Autodesk Inventor part; units mm, degrees
ref_plane "YZ Plane" through (0, 0, 0) normal (1, 0, 0) x (0, 1, 0)
ref_plane "XZ Plane" through (0, 0, 0) normal (0, 1, 0) x (-1, 0, 0)
ref_plane "XY Plane" through (0, 0, 0) normal (0, 0, 1) x (1, 0, 0)
sketch "Sketch1" plane through (0, 0, 0) normal (0, 1, 0) x (-1, 0, 0)
  line L0 (0, 0) -> (0, -11.938)
  line L1 (-15.24, 3.3655) -> (-15.24, -15.3035)
  line L2 (0, 0) -> (-15.24, 3.3655)
  line L3 (0, -11.938) -> (-15.24, -15.3035)
  line L4 (-15.24, 3.3655) -> (-19.05, 3.3655)
  line L5 (-19.05, 3.3655) -> (-19.05, 2.0955)
  line L6 (-19.05, 2.0955) -> (-15.24, 2.0955)
  line L7 (-15.24, 2.0955) -> (-15.24, 3.3655)
  line L8 (-15.24, -15.3035) -> (-19.05, -15.3035)
  line L9 (-19.05, -15.3035) -> (-19.05, -14.0335)
  line L10 (-19.05, -14.0335) -> (-15.24, -14.0335)
  line L11 (-15.24, -14.0335) -> (-15.24, -15.3035)
  line L12 (0, 0) -> (0, 3.175)
  line L13 (-15.24, 3.3655) -> (-15.24, 6.5405)
  line L14 (0, -11.938) -> (0, -15.113)
  line L15 (-15.24, -15.3035) -> (-15.24, -18.4785)
  line L16 (-15.24, -18.4785) -> (0, -15.113)
  line L17 (0, 3.175) -> (-15.24, 6.5405)
  line L18 (-15.24, 6.5405) -> (-34.29, 6.5405)
  line L19 (-19.05, 3.3655) -> (-34.29, 3.3655)
  line L20 (-34.29, 3.3655) -> (-34.29, 6.5405)
  line L21 (-15.24, -18.4785) -> (-34.29, -18.4785)
  line L22 (-34.29, -18.4785) -> (-34.29, -15.3035)
  line L23 (-34.29, -15.3035) -> (-19.05, -15.3035)
  line L24 (-34.29, 6.5405) -> (-37.465, 6.5405)
  line L25 (-37.465, 6.5405) -> (-37.465, -18.4785)
  line L26 (-37.465, -18.4785) -> (-34.29, -18.4785)
  line L27 (-34.29, -18.4785) -> (-34.29, 6.5405)
  line L28 (-15.24, -15.3035) -> (-34.29, -15.3035)
  line L29 (-34.29, -15.3035) -> (-34.29, 3.3655)
  line L30 (-34.29, 3.3655) -> (-15.24, 3.3655)
  line L31 (-15.24, 3.3655) -> (-15.24, -15.3035)
  line L32 (-15.24, 3.3655) -> (-34.29, 3.3655)
  line L33 (-34.29, 3.3655) -> (-34.29, 6.5405)
  line L34 (-34.29, 6.5405) -> (-15.24, 6.5405)
  line L35 (-15.24, 6.5405) -> (-15.24, 3.3655)
  dimension "d0" = 11.938
  dimension "d1" = 15.24
  dimension "d2" = 18.669
  dimension "d3" = 3.3655
  dimension "d4" = 3.81
  dimension "d5" = 1.27
  dimension "d6" = 3.81
  dimension "d7" = 1.27
  dimension "d8" = 3.175
  dimension "d9" = 3.175
  dimension "d10" = 3.175
  dimension "d11" = 3.175
  dimension "d12" = 19.05
  dimension "d13" = 3.175
extrude "Extrusion4" add sketch "Sketch1" along normal blind 1.5875
sketch "Sketch4" plane through (0, 1.5875, 0) normal (0, 1, 0) x (1, 0, 0)
  circle A0 centre (8.636, 5.969) radius 1.5875
  line L0 (0, 15.113) -> (0, -3.175)
  point P0 (0, 0)
  dimension "d26" = 3.175
  dimension "d27" = 8.636
extrude "Extrusion5" cut sketch "Sketch4" against normal blind 1.5875
chamfer "Chamfer2" distance 1.27 angle 45 1 edges at (7.0485, 0, -5.969)
equation "\"d3\" = -0.5 * d0 + 0.5 * d2"
properties part number "phototransistorMount2" material "ABS Plastic"
Input: part model. Units: mm. Frame: model coordinates. Round coordinates to 2 decimals unless told otherwise and drop trailing zeros. Loops run counter-clockwise (first coordinate to the right, second up) from the corner with the lowest first, then second, coordinate; pieces in that order, holes last. Notation, with made-up numbers: M 63.25,86.5 L 95.25,86.5 A16 cw 95.25,100.5 Z; hole C 43.5,33.5 d10. An arc over 180 degrees is marked long. Answer in a Markdown table with one row per item. Add a question column.
1. Section C-C (x = 12). Output: boundary loops of the cut face in (y, z) (1 decimal), and give its area (3 significant figures).
2. Mould query, pull axis Z, two halves, no side actions, for faces 1 (the face through (26, 1, 6.54)), 2 (the face through (26, 1, -18.478)), 3 (the face through (7.466, 1.431, -7.042)). Classes: released by +Z, released by -Z, zero draft, split by the parting line, or undercut.
3. Contact query for a flat-ended pin moving along its axis: pin 1 (3.5 mm diameter, centred on x = 8.636, z = -5.969, fed in from -Y). Output: stop coordinate, or through.
4. Section A-A (y = 0.8). Output: boundary loops of the cut face in (x, z) (1 decimal), and give its area (3 significant figures).
5. Ray query, probe 1 along Z at (x, y) = (9.5, 1.1); probe 2 along Z at (x, y) = (6.5, 0.3); probe 3 along Z at (x, y) = (2.5, 1.45). Return the intervals inside material, ascending.
6. Section B-B (x = 3.5). Output: boundary loops of the cut face in (y, z), and give its area (3 significant figures).
Values follow:
| question | item | result |
|---|---|---|
| 1 | outline | M 0,-17.8 L 1.6,-17.8 L 1.6,5.8 L 0,5.8 Z |
| 1 | area | 37.4 mm^2 |
| 2 | face 1 | released by +Z |
| 2 | face 2 | released by -Z |
| 2 | face 3 | undercut |
| 3 | pin 1 | y = 1.11 |
| 4 | outline | M 0,-15.1 L 15.2,-18.5 L 37.5,-18.5 L 37.5,6.5 L 15.2,6.5 L 0,3.2 Z; hole C 8.6,-6 d4.1 |
| 4 | area | 873 mm^2 |
| 5 | probe 1 | -17.21 to -7.5, -4.44 to 5.27 |
| 5 | probe 2 | -16.55 to -7.38, -4.56 to 4.61 |
| 5 | probe 3 | -15.67 to 3.73 |
| 6 | outline | M 0,-15.89 L 1.59,-15.89 L 1.59,3.95 L 0,3.95 Z |
| 6 | area | 31.5 mm^2 |
